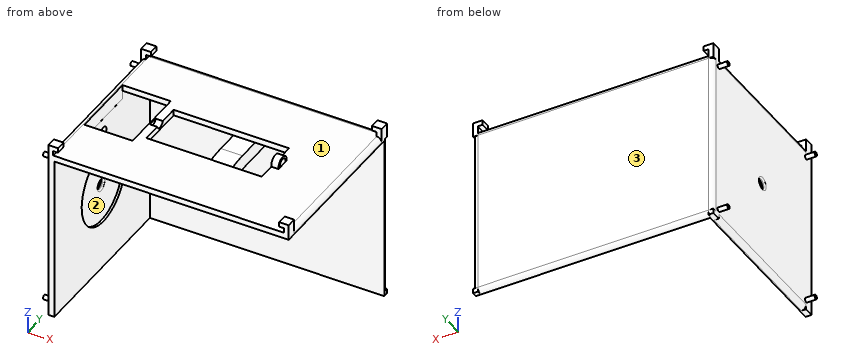
```python
from build123d import *

# Parameters (mm, degrees)
SKETCH1_W            = 127
SKETCH1_H            = 91.44
BOSS_EXTRUDE1_DEPTH  = 228.6
SKETCH3_W            = 120.65
SKETCH3_H            = 85.09
CUT_EXTRUDE1_DEPTH   = 226.06
SKETCH2_R            = 2.667
CUT_EXTRUDE2_DEPTH   = 266.475570251
SKETCH4_R            = 1.143
BOSS_EXTRUDE3_DEPTH  = 5.08
SKETCH5_R            = 20.32
CUT_EXTRUDE3_DEPTH   = 1.27
FILLET1_R            = 0.762
FILLET2_R            = 0.762
FILLET3_R            = 0.762
SKETCH6_W            = 60.96
SKETCH6_H            = 25.4
CUT_EXTRUDE4_DEPTH   = 256.582569828
FILLET4_R            = 2.54
SKETCH7_W            = 85.09
SKETCH7_H            = 111.152565629
CUT_EXTRUDE5_DEPTH   = 268.942913323
SKETCH10_R           = 2.667
CUT_EXTRUDE6_DEPTH   = 2.54
CUT_EXTRUDE7_DEPTH   = 7.62
SKETCH13_R           = 2.667
CUT_EXTRUDE8_DEPTH   = 2.54
CUT_EXTRUDE9_DEPTH   = 7.62
SKETCH20_W           = 11.43
SKETCH20_H           = 7.62
BOSS_EXTRUDE4_DEPTH  = 50.8
CUT_EXTRUDE10_START  = -12.7
SKETCH21_R           = 2.667
CUT_EXTRUDE10_DEPTH  = 12.7
CUT_EXTRUDE11_DEPTH  = 12.7
SKETCH24_R           = 3.81
BOSS_EXTRUDE5_DEPTH  = 3.81
SKETCH25_R           = 2.667
CUT_EXTRUDE12_DEPTH  = 3.81
CUT_EXTRUDE13_DEPTH  = 12.7
CUT_EXTRUDE14_START  = 64.77
SKETCH27_R           = 2.667
CUT_EXTRUDE14_DEPTH  = 64.77
CUT_EXTRUDE15_START  = 64.77
SKETCH29_R           = 2.667
CUT_EXTRUDE15_DEPTH  = 64.77
FILLET6_R            = 50.8
FILLET7_R            = 50.8
BOSS_EXTRUDE6_DEPTH  = 5.08
MIRROR5_COPY_1_DEPTH = 5.08
MIRROR6_COPY_1_DEPTH = 5.08
MIRROR6_COPY_2_DEPTH = 5.08
MIRROR6_COPY_3_DEPTH = 5.08
SKETCH35_W           = 127
SKETCH35_H           = 137.16
CUT_EXTRUDE16_DEPTH  = 52.07
SKETCH39_W           = 85.09
SKETCH39_H           = 88.9
CUT_EXTRUDE20_DEPTH  = 52.07
SKETCH41_W           = 123.825
SKETCH41_H           = 88.9
CUT_EXTRUDE21_DEPTH  = 52.07
SKETCH42_W           = 127
SKETCH42_H           = 5.08
CUT_EXTRUDE22_DEPTH  = 236.22


with BuildPart() as part:
    # Sketch1 → Boss-Extrude1 (new body)
    with BuildSketch(Plane(origin=(0, 0, 0), x_dir=(1, 0, 0), z_dir=(0, 1, 0))):
        Rectangle(SKETCH1_W, SKETCH1_H)
    extrude(amount=BOSS_EXTRUDE1_DEPTH)

    # Sketch3 → Cut-Extrude1 (cut)
    with BuildSketch(Plane.XZ):
        Rectangle(SKETCH3_W, SKETCH3_H)
    extrude(amount=-CUT_EXTRUDE1_DEPTH, mode=Mode.SUBTRACT)

    # Sketch2 → Cut-Extrude2 (cut, through all)
    with BuildSketch(Plane(origin=(63.5, 0, 0), x_dir=(0, 0, -1), z_dir=(1, 0, 0))):
        with Locations((0, 182.88)):
            Circle(SKETCH2_R)
    extrude(amount=-CUT_EXTRUDE2_DEPTH, mode=Mode.SUBTRACT)

    # Sketch4 → Boss-Extrude3 (add)
    with BuildSketch(Plane(origin=(63.5, 0, 0), x_dir=(0, 0, -1), z_dir=(1, 0, 0))):
        with Locations(Location((-40.64, 223.52, 0), (0, 0, 180))):
            Circle(SKETCH4_R)
        with Locations(Location((40.64, 223.52, 0), (0, 0, 180))):
            Circle(SKETCH4_R)
        with Locations(Location((40.64, 142.24, 0), (0, 0, 180))):
            Circle(SKETCH4_R)
        with Locations(Location((-40.64, 142.24, 0), (0, 0, 180))):
            Circle(SKETCH4_R)
    boss_extrude3 = extrude(amount=BOSS_EXTRUDE3_DEPTH)

    # Sketch5 → Cut-Extrude3 (cut)
    with BuildSketch(Plane.ZY.offset(-60.325)):
        with Locations((0, 182.88)):
            Circle(SKETCH5_R)
    cut_extrude3 = extrude(amount=-CUT_EXTRUDE3_DEPTH, mode=Mode.SUBTRACT)

    # Fillet1
    fillet1_edges = [part.edges().sort_by_distance(p)[0] for p in [
        (61.595, 182.88, 2.667),
    ]]
    fillet(fillet1_edges, radius=FILLET1_R)

    # Fillet2
    fillet2_edges = [part.edges().sort_by_distance(p)[0] for p in [
        (63.5, 182.88, 2.667),
    ]]
    fillet(fillet2_edges, radius=FILLET2_R)

    # Mirror2: Boss-Extrude3, Cut-Extrude3 across plane
    add(boss_extrude3.mirror(Plane(origin=(0, 0, 0), x_dir=(0, 0, 1), z_dir=(1, 0, 0))))
    add(cut_extrude3.mirror(Plane(origin=(0, 0, 0), x_dir=(0, 0, 1), z_dir=(1, 0, 0))), mode=Mode.SUBTRACT)

    # Fillet3
    fillet3_edges = [part.edges().sort_by_distance(p)[0] for p in [
        (-63.5, 182.88, 2.667),
        (-61.595, 182.88, 2.667),
    ]]
    fillet(fillet3_edges, radius=FILLET3_R)

    # Sketch6 → Cut-Extrude4 (cut, through all)
    with BuildSketch(Plane.XY.offset(45.72)):
        with Locations((0, 182.88)):
            Rectangle(SKETCH6_W, SKETCH6_H)
    extrude(amount=-CUT_EXTRUDE4_DEPTH, mode=Mode.SUBTRACT)

    # Fillet4
    fillet4_edges = [part.edges().sort_by_distance(p)[0] for p in [
        (-63.5, 228.6, 0),
        (0, 228.6, 45.72),
        (63.5, 228.6, 0),
        (63.5, 114.3, 45.72),
        (-63.5, 114.3, 45.72),
        (-63.5, 114.3, -45.72),
        (63.5, 114.3, -45.72),
        (0, 228.6, -45.72),
    ]]
    fillet(fillet4_edges, radius=FILLET4_R)

    # Sketch7 → Cut-Extrude5 (cut, through all)
    with BuildSketch(Plane(origin=(63.5, 0, 0), x_dir=(0, 0, -1), z_dir=(1, 0, 0))):
        with Locations((0, 75.896282814)):
            Rectangle(SKETCH7_W, SKETCH7_H)
    extrude(amount=-CUT_EXTRUDE5_DEPTH, mode=Mode.SUBTRACT)

    # Sketch10 → Cut-Extrude6 (cut)
    with BuildSketch(Plane.ZY.offset(-60.325)):
        with Locations((-30.48, 182.88)):
            Circle(SKETCH10_R)
    extrude(amount=-CUT_EXTRUDE6_DEPTH, mode=Mode.SUBTRACT)

    # Sketch12 → Cut-Extrude7 (cut)
    with BuildSketch(Plane(origin=(0, 0, -45.72), x_dir=(-1, 0, 0), z_dir=(0, 0, -1))):
        Polygon((-34.810362372, 182.807903476), (-34.810362372, 200.587903476), (-60.210362372, 200.587903476), (-60.210362372, 182.807903476), (-60.210362372, 165.027903476), (-34.810362372, 165.027903476), align=None)
    extrude(amount=-CUT_EXTRUDE7_DEPTH, mode=Mode.SUBTRACT)

    # Sketch13 → Cut-Extrude8 (cut)
    with BuildSketch(Plane(origin=(-60.325, 0, 0), x_dir=(0, 0, -1), z_dir=(1, 0, 0))):
        with Locations((-30.48, 182.88)):
            Circle(SKETCH13_R)
    extrude(amount=-CUT_EXTRUDE8_DEPTH, mode=Mode.SUBTRACT)

    # Sketch16 → Cut-Extrude9 (cut)
    with BuildSketch(Plane.XY.offset(45.72)):
        Polygon((-60.34639287, 182.934228321), (-60.34639287, 200.714228321), (-34.94639287, 200.714228321), (-34.94639287, 165.154228321), (-60.34639287, 165.154228321), align=None)
    extrude(amount=-CUT_EXTRUDE9_DEPTH, mode=Mode.SUBTRACT)

    # Sketch20 → Boss-Extrude4 (add)
    with BuildSketch(Plane.XZ.offset(-226.06)):
        with Locations((1.27, -30.48)):
            Rectangle(SKETCH20_W, SKETCH20_H)
    boss_extrude4 = extrude(amount=BOSS_EXTRUDE4_DEPTH)

    # Sketch21 → Cut-Extrude10 (cut)
    with BuildSketch(Plane(origin=(6.985, 0, 0), x_dir=(0, 0, -1), z_dir=(1, 0, 0)).offset(CUT_EXTRUDE10_START)):
        with Locations(Location((30.48, 182.88, 0), (0, 0, 180))):
            Circle(SKETCH21_R)
    cut_extrude10 = extrude(amount=CUT_EXTRUDE10_DEPTH, mode=Mode.SUBTRACT)

    # Sketch23 → Cut-Extrude11 (cut)
    with BuildSketch(Plane(origin=(6.985, 0, 0), x_dir=(0, 0, -1), z_dir=(1, 0, 0))):
        Polygon((27.813, 182.88), (26.67, 182.88), (26.67, 175.26), (34.29, 175.26), (34.29, 182.88), align=None)
    extrude(amount=-CUT_EXTRUDE11_DEPTH, mode=Mode.SUBTRACT)

    # Sketch24 → Boss-Extrude5 (add)
    with BuildSketch(Plane.ZY.offset(-30.48)):
        with Locations((-46.355, 182.88)):
            Circle(SKETCH24_R)
    boss_extrude5 = extrude(amount=-BOSS_EXTRUDE5_DEPTH)

    # Sketch25 → Cut-Extrude12 (cut)
    with BuildSketch(Plane.ZY.offset(-30.48)):
        with Locations((-46.355, 182.88)):
            Circle(SKETCH25_R)
    cut_extrude12 = extrude(amount=-CUT_EXTRUDE12_DEPTH, mode=Mode.SUBTRACT)

    # Mirror3: Boss-Extrude4, Cut-Extrude10, Boss-Extrude5, Cut-Extrude12 across plane
    add(boss_extrude4.mirror(Plane.XY))
    add(cut_extrude10.mirror(Plane.XY), mode=Mode.SUBTRACT)
    add(boss_extrude5.mirror(Plane.XY))
    add(cut_extrude12.mirror(Plane.XY), mode=Mode.SUBTRACT)

    # Sketch26 → Cut-Extrude13 (cut)
    with BuildSketch(Plane(origin=(6.985, 0, 0), x_dir=(0, 0, -1), z_dir=(1, 0, 0))):
        Polygon((-27.813, 182.88), (-26.67, 182.88), (-26.67, 175.26), (-34.29, 175.26), (-34.29, 182.88), align=None)
    extrude(amount=-CUT_EXTRUDE13_DEPTH, mode=Mode.SUBTRACT)

    # Sketch27 → Cut-Extrude14 (cut)
    with BuildSketch(Plane.ZY.offset(-30.48).offset(CUT_EXTRUDE14_START)):
        with Locations((-46.355, 182.88)):
            Circle(SKETCH27_R)
    extrude(amount=-CUT_EXTRUDE14_DEPTH, mode=Mode.SUBTRACT)

    # Sketch29 → Cut-Extrude15 (cut)
    with BuildSketch(Plane.ZY.offset(-30.48).offset(CUT_EXTRUDE15_START)):
        with Locations(Location((46.355, 182.88, 0), (0, 0, 256.225853002))):
            Circle(SKETCH29_R)
    extrude(amount=-CUT_EXTRUDE15_DEPTH, mode=Mode.SUBTRACT)

    # Fillet6
    # the kernel refuses this fillet: 50.8 mm, written as the material it takes off along each edge
    with BuildSketch(Plane(origin=(33.773797915, 182.88, 34.29), x_dir=(0, 0, -1), z_dir=(-1, 0, 0))) as fillet6_piece_1:
        with BuildLine():
            CenterArc((50.8, -10.715519166), FILLET6_R, 167.822824326, 12.177175674)
            Line((0, -10.715519166), (-1.016, -10.715519166))
            Line((-1.016, -10.715519166), (-1.016, 0))
            Line((-1.016, 0), (0, 1.016))
            ThreePointArc((0, 1.016), (0.5715, 1.016), (0.14986, 0.214310383))
            Line((0.14986, 0.214310383), (1.143, 0))
        make_face()
    extrude(amount=65.007595831, mode=Mode.SUBTRACT)

    # Fillet7
    # the kernel refuses this fillet: 50.8 mm, written as the material it takes off along each edge
    with BuildSketch(Plane(origin=(33.773797915, 182.88, -34.29), x_dir=(0, 1, 0), z_dir=(-1, 0, 0))) as fillet7_piece_1:
        with BuildLine():
            CenterArc((10.715519166, -50.8), FILLET7_R, 90, 12.177175674)
            Line((0, -1.143), (0, 0))
            Line((0, 0), (10.715519166, 0))
        make_face()
    extrude(amount=65.007595831, mode=Mode.SUBTRACT)

    # Sketch33 → Boss-Extrude6 (add)
    with BuildSketch(Plane(origin=(0, 228.6, 0), x_dir=(1, 0, 0), z_dir=(0, 1, 0))):
        Polygon((63.5, 43.18), (63.5, 50.8), (58.42, 50.8), (58.42, 48.26), (60.96, 48.26), (60.96, 43.18), align=None)
    boss_extrude6 = extrude(amount=-BOSS_EXTRUDE6_DEPTH)

    # Mirror4: Boss-Extrude6 across plane
    add(boss_extrude6.mirror(Plane(origin=(0, 0, 0), x_dir=(0, 0, 1), z_dir=(1, 0, 0))))

    # Mirror5: Boss-Extrude6 across plane
    add(boss_extrude6.mirror(Plane.ZX.offset(182.88)))

    # Mirror5 copy 1 sketch → Mirror5 copy 1 (add)
    with BuildSketch(Plane(origin=(0, 137.16, 0), x_dir=(-1, 0, 0), z_dir=(0, -1, 0))):
        Polygon((63.5, 43.18), (63.5, 50.8), (58.42, 50.8), (58.42, 48.26), (60.96, 48.26), (60.96, 43.18), align=None)
    extrude(amount=-MIRROR5_COPY_1_DEPTH)

    # Mirror6: Boss-Extrude6 across plane
    add(boss_extrude6.mirror(Plane.XY))

    # Mirror6 copy 1 sketch → Mirror6 copy 1 (add)
    with BuildSketch(Plane(origin=(0, 228.6, 0), x_dir=(-1, 0, 0), z_dir=(0, 1, 0))):
        Polygon((63.5, 43.18), (63.5, 50.8), (58.42, 50.8), (58.42, 48.26), (60.96, 48.26), (60.96, 43.18), align=None)
    extrude(amount=-MIRROR6_COPY_1_DEPTH)

    # Mirror6 copy 2 sketch → Mirror6 copy 2 (add)
    with BuildSketch(Plane.XZ.offset(-137.16)):
        Polygon((63.5, 43.18), (63.5, 50.8), (58.42, 50.8), (58.42, 48.26), (60.96, 48.26), (60.96, 43.18), align=None)
    extrude(amount=-MIRROR6_COPY_2_DEPTH)

    # Mirror6 copy 3 sketch → Mirror6 copy 3 (add)
    with BuildSketch(Plane(origin=(0, 137.16, 0), x_dir=(-1, 0, 0), z_dir=(0, -1, 0))):
        Polygon((63.5, -43.18), (63.5, -50.8), (58.42, -50.8), (58.42, -48.26), (60.96, -48.26), (60.96, -43.18), align=None)
    extrude(amount=-MIRROR6_COPY_3_DEPTH)

    # Sketch35 → Cut-Extrude16 (cut, symmetric)
    with BuildSketch(Plane.XY):
        with Locations((0, 68.58)):
            Rectangle(SKETCH35_W, SKETCH35_H)
    extrude(amount=CUT_EXTRUDE16_DEPTH, both=True, mode=Mode.SUBTRACT)

    # Sketch39 → Cut-Extrude20 (cut, symmetric)
    with BuildSketch(Plane(origin=(63.5, 0, 0), x_dir=(0, 0, -1), z_dir=(1, 0, 0))):
        with Locations((0, 181.61)):
            Rectangle(SKETCH39_W, SKETCH39_H)
    extrude(amount=CUT_EXTRUDE20_DEPTH, both=True, mode=Mode.SUBTRACT)

    # Sketch41 → Cut-Extrude21 (cut, symmetric)
    with BuildSketch(Plane(origin=(0, 0, -45.72), x_dir=(-1, 0, 0), z_dir=(0, 0, -1))):
        with Locations((-1.5875, 181.61)):
            Rectangle(SKETCH41_W, SKETCH41_H)
    extrude(amount=CUT_EXTRUDE21_DEPTH, both=True, mode=Mode.SUBTRACT)

    # Sketch42 → Cut-Extrude22 (cut)
    with BuildSketch(Plane(origin=(0, 0, 0), x_dir=(1, 0, 0), z_dir=(0, 1, 0))):
        with Locations((0, 48.26)):
            Rectangle(SKETCH42_W, SKETCH42_H)
    extrude(amount=CUT_EXTRUDE22_DEPTH, mode=Mode.SUBTRACT)


solid = part.part
```
Can you work these out from the model? Positions are in its coordinate system, mm. Face numbers are marked on the shaded views. Coordinates: 2 decimals unless noted, no trailing zeros. Loops run counter-clockwise (first coordinate to the right, second up) from the corner with the lowest first, then second, coordinate; pieces in that order, holes last.
1) For pin 1 (4 mm diameter, centred on y = 213.5, z = 25, fed in from -X); pin 2 (5.5 mm diameter, centred on x = 0, y = 198, fed in from -Z); pin 3 (12 mm diameter, centred on x = 43.5, y = 162, fed in from +Z); pin 4 (2.5 mm diameter, centred on y = 187.5, z = 42.5, fed in from +X), each with a flat end and sliding along its axis, tell me the tip position at first contact or that it passes through.
2) I need wall thicknesses on probe 1 along Z at (x, y) = (-62.45, 182.88); probe 2 along Z at (x, y) = (-61.95, 182.88); probe 3 along X at (y, z) = (188, -25) (3 decimals). Which ranges of each line are inside material? Lowest first, please.
3) Imagine slicing it at C-C on z = 0. List the corners of the cut face in (x, y) for me (3 decimals), plus the area to 3 significant figures.
4) Thinking about a two-plate mould opening in Y: for the marked faces 1, 2 and 3, which applies, pulls with the +Y half, pulls with the -Y half, needs draft (parallel to the pull), parting line crosses it, or undercut?
5) Imagine slicing it at D-D on y = 157. List the corners of the cut face in (x, z) for me (3 decimals).
6) Imagine slicing it at B-B on x = -55. List the corners of the cut face in (y, z) for me (3 decimals), plus the area to 3 significant figures.
7) Imagine slicing it at A-A on y = 208. List the corners of the cut face in (x, z) for me (3 decimals).
Completed:
1. pin 1: stops at x = -63.5
1. pin 2: stops at z = 26.67
1. pin 3: stops at z = 45.72
1. pin 4: stops at x = 63.5
2. probe 1: z = -45.24 to -2.67, 2.67 to 27.81, 33.15 to 45.24
2. probe 2: z = -45.52 to -2.78, 2.78 to 27.81, 33.15 to 45.52
2. probe 3: x = -63.5 to -60.325
3. outline: (-63.5, 137.16) - (-60.325, 137.16) - (-60.325, 162.56) - (-61.595, 162.56) - (-61.595, 179.451) arc R0.762 ccw to (-62.357, 180.213) - (-62.738, 180.213) arc R0.762 ccw to (-63.5, 179.451) - close; (-63.5, 186.309) arc R0.762 ccw to (-62.738, 185.547) - (-62.357, 185.547) arc R0.762 ccw to (-61.595, 186.309) - (-61.595, 203.2) - (-60.325, 203.2) - (-60.325, 226.06) - (63.5, 226.06) arc R2.54 ccw to (60.96, 228.6) - (-60.96, 228.6) arc R2.54 ccw to (-63.5, 226.06) - close
3. area: 540 mm2
4. face 1: needs draft
4. face 2: undercut
4. face 3: pulls with the +Y half
5. outline: (-63.5, -43.18) arc R2.54 ccw to (-60.96, -45.72) - (-60.325, -45.72) - (-60.325, 42.545) - (63.5, 42.545) - (63.5, 43.18) arc R2.54 ccw to (60.96, 45.72) - (-60.96, 45.72) arc R2.54 ccw to (-63.5, 43.18) - close
6. outline: (137.16, 42.545) - (165.154, 42.545) - (165.154, 45.72) - (137.16, 45.72) - close; (200.714, 42.545) - (226.06, 42.545) - (226.06, -45.72) arc R2.54 ccw to (228.6, -43.18) - (228.6, 43.18) arc R2.54 ccw to (226.06, 45.72) - (200.714, 45.72) - close
6. area: 399 mm2
7. outline: (-63.5, -43.18) arc R2.54 ccw to (-60.96, -45.72) - (-60.325, -45.72) - (-60.325, 42.545) - (63.5, 42.545) - (63.5, 43.18) arc R2.54 ccw to (60.96, 45.72) - (-60.96, 45.72) arc R2.54 ccw to (-63.5, 43.18) - close; (-4.445, 26.67) - (6.985, 26.67) - (6.985, 34.29) - (-4.445, 34.29) - close
